```python
from build123d import *

# Parameters (mm, degrees)
CHAMFER1_SIZE      = 0.29
CHAMFER1_SIZE2     = 0.502294734
CUT_EXTRUDE1_DEPTH = 1.58
DRAFT1_ANGLE       = -35
DRAFT2_ANGLE       = -8
FILLET1_R          = 0.25


with BuildPart() as part:
    # Sketch1 → Revolve1 (revolve)
    with BuildSketch(Plane.XY, mode=Mode.PRIVATE) as revolve1_sk:
        with BuildLine():
            Line((0, 3.75), (0, 1.45))
            Line((0, 1.45), (6.5, 1.45))
            Line((6.5, 1.45), (6.5, 0))
            Line((6.5, 0), (-2.35, 0))
            ThreePointArc((-2.35, 0), (-1.940427702, 1.71610023), (-0.8, 3.0622704))
            Line((-0.8, 3.0622704), (-0.8, 3.75))
            Line((-0.8, 3.75), (0, 3.75))
        make_face()
    revolve(revolve1_sk.sketch.rotate(Axis((-6.478309986, 0, 0), (1, 0, 0)), 90), axis=Axis((-6.478309986, 0, 0), (1, 0, 0)))

    # Chamfer1
    chamfer1_edges = [part.edges().sort_by_distance(p)[0] for p in [
        (6.5, 0, -1.45),
    ]]
    chamfer1_side = [part.faces().sort_by_distance(p)[0] for p in [
        (6.5, 0, 0),
    ]]
    chamfer(chamfer1_edges, length=CHAMFER1_SIZE, length2=CHAMFER1_SIZE2, reference=chamfer1_side[0])

    # Sketch4 → Cut-Extrude1 (cut)
    with BuildSketch(Plane(origin=(-2.35, 0, 0), x_dir=(0, 0, -1), z_dir=(1, 0, 0))):
        Polygon((0.3, 1.5), (-0.3, 1.5), (-0.3, 0.3), (-1.5, 0.3), (-1.5, -0.3), (-0.3, -0.3), (-0.3, -1.5), (0.3, -1.5), (0.3, -0.3), (1.5, -0.3), (1.5, 0.3), (0.3, 0.3), align=None)
    extrude(amount=CUT_EXTRUDE1_DEPTH, mode=Mode.SUBTRACT)

    # Draft1
    draft1_faces = [part.faces().sort_by_distance(p)[0] for p in [
        (-1.403564361, 0, -1.5),
        (-1.403564361, -1.5, 0),
        (-1.403564361, 0, 1.5),
        (-1.403564361, 1.5, 0),
    ]]
    draft(draft1_faces, Plane.YZ.offset(-2.35), DRAFT1_ANGLE)

    # Draft2
    draft2_faces = [part.faces().sort_by_distance(p)[0] for p in [
        (-1.709589538, 0.648659775, -0.3),
        (-1.709589538, 0.3, -0.648659775),
        (-1.709589538, -0.3, -0.648659775),
        (-1.709589538, -0.648659775, -0.3),
        (-1.709589538, -0.648659775, 0.3),
        (-1.709589538, -0.3, 0.648659775),
        (-1.709589538, 0.3, 0.648659775),
        (-1.709589538, 0.648659775, 0.3),
    ]]
    draft(draft2_faces, Plane.YZ.offset(-2.35), DRAFT2_ANGLE)

    # Fillet1
    fillet1_edges = [part.edges().sort_by_distance(p)[0] for p in [
        (-1.548378832, 0.187339492, -0.187339492),
        (-1.548378832, 0.187339492, 0.187339492),
        (-1.548378832, -0.187339492, 0.187339492),
        (-1.548378832, -0.187339492, -0.187339492),
    ]]
    fillet(fillet1_edges, radius=FILLET1_R)


solid = part.part
```
Read the model definition and answer for the solid it produces. Units are mm, in the model's axes. A direction names the side the tool comes from. Give positions to 0.01 mm unless a question says otherwise; leave off trailing zeros. Write each loop counter-clockwise with the first axis right and the second up, starting at its lowest first coordinate (ties: lowest second). Pieces come first, ordered by that corner, then holes. Notation, with made-up numbers: (18.25, 64) -> (30.25, 64) arc R20 ccw to (30.25, 75) -> close; hole circle Ø7 at (87, 15). An arc over 180 degrees is marked (long way). Answer as a JSON object with one key per item and string values.
1) Flat-ended cylindrical pins translate along their axes: pin 1 Ø1.5 at (x, y) = (1.5, -2) entering from +Z; pin 2 Ø2 at (x, y) = (3, -1.5) entering from +Z; pin 3 Ø3 at (x, y) = (2.5, 2.5) entering from +Z. Find the tip coordinate at first contact, or state that the pin passes through.
Findings below:
{"pin 1": "stops at z = 0.73", "pin 2": "stops at z = 1.36", "pin 3": "stops at z = 1.05"}
2) Section C-C on y = -2 is taken. Write down the section's boundary in (x, z).
Findings below:
{"outline": "(-0.8, -3.17) -> (0, -3.17) -> (0, 3.17) -> (-0.8, 3.17) -> (-0.8, 2.32) arc R3.23 ccw to (-0.8, -2.32) -> close"}
3) Straight lines are drawn through the part: probe 1 along X at (y, z) = (-1, 3.25); probe 2 along Z at (x, y) = (-1.5, -0.25); probe 3 along X at (y, z) = (3, 0.25). For each, find the intervals that lie inside material, in ascending order. Write a range as from..to.
Findings below:
{"probe 1": "x = -0.8..0", "probe 2": "z = -2.38..-0.26, 0.26..2.38", "probe 3": "x = -0.87..0"}
4) For a pull along Y with two mould halves and no side action, classify faces 1 (the flat face through (-1.72, 0.21, -0.72)), 2 (the flat face through (6.5, 0, 0)), 3 (the cylindrical face through (3.04, -0.06, -1.45)) as pulls with the +Y half, pulls with the -Y half, needs draft (parallel to the pull), parting line crosses it, or undercut.
Findings below:
{"face 1": "undercut", "face 2": "needs draft", "face 3": "parting line crosses it"}
5) Section A-A on x = -0.5 is taken. Write down the section's boundary in (y, z), then the cut area to 3 significant figures.
Findings below:
{"outline": "circle Ø7.5 at (0, 0)", "area": "44.2 mm^2"}
6) A tool of negligible diameter and unlimited length cuts with its end or side. For faces 4 (the cylindrical face through (-0.39, -3.16, 2.02)), 5 (the flat face through (0, 2, 0)), 6 (the flat face through (-1.598, 0.973, -0.004)), from which of +Z, -Z, +X, -X, +Y, -Y can it reach the whole face along a straight path? Write none if from no direction.
Findings below:
{"face 4": "+X, -X", "face 5": "+X", "face 6": "-X"}
7) Section D-D on x = 1.5 is taken. Write down the section's boundary in (y, z).
Findings below:
{"outline": "circle Ø2.9 at (0, 0)"}
